from build123d import *

# Parameters (mm, degrees)
BOSS_EXTRUDE1_DEPTH = 3
CIRPATTERN1_COUNT   = 8


with BuildPart() as part:
    # Sketch1 → Boss-Extrude1 (new body)
    with BuildSketch(Plane(origin=(0, 0, 0), x_dir=(1, 0, 0), z_dir=(0, 1, 0))):
        Polygon((0, 0), (105.018289963, 0), (105.018289963, 43.5), (74.259144982, 74.259144982), align=None)
    boss_extrude1 = extrude(amount=BOSS_EXTRUDE1_DEPTH)

    # CirPattern1: Boss-Extrude1 ×8 about axis
    cirpattern1_axis = Axis((0, 0, 0), (0, 1, 0))
    for i in range(1, CIRPATTERN1_COUNT):
        add(boss_extrude1.rotate(cirpattern1_axis, i * 360 / CIRPATTERN1_COUNT))


solid = part.part
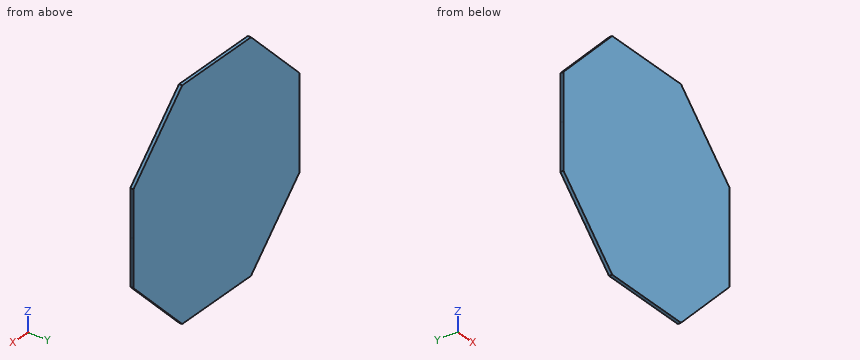
Could you check a few things on this model? Use its own coordinates, in mm. Give positions to 0.01 mm unless a question says otherwise; leave off trailing zeros. Order: outer loops, then holes, each group sorted by start corner. A loop starts at its lowest first (then second) coordinate and runs counter-clockwise, first axis right, second up.
1. Suppose I cut it at B-B (z = -91). List the corners of the cut face in (x, y) for me.
2. Suppose I cut it at C-C (x = -81.5). List the corners of the cut face in (y, z) for me.
3. Suppose I cut it at A-A (y = 1.35). List the corners of the cut face in (x, z) for me, plus the area to 3 significant figures.
4. I need wall thicknesses on L1, parallel to X at y = 2, z = 45.5; L2, parallel to X at y = 1.75, z = -45; L3, parallel to Z at x = -89, y = 2.8. Which ranges of each line are inside material? Lowest first, please.
5. Will this pin go through, and if not, where does the flat tip stop? P1, Ø6, axis at x = -71.5, z = -75.5, coming from the -Y side.
Solved:
1. outline: (-57.52, 0) - (57.52, 0) - (57.52, 3) - (-57.52, 3) - close
2. outline: (0, -67.02) - (3, -67.02) - (3, 67.02) - (0, 67.02) - close
3. outline: (-105.02, -43.5) - (-43.5, -105.02) - (43.5, -105.02) - (105.02, -43.5) - (105.02, 43.5) - (43.5, 105.02) - (-43.5, 105.02) - (-105.02, 43.5) - close
3. area: 36,500 mm2
4. L1: x = -103.02 to 103.02
4. L2: x = -103.52 to 103.52
4. L3: z = -59.52 to 59.52
5. P1: stops at y = 0
